from build123d import *
from OCP.BRepFilletAPI import BRepFilletAPI_MakeChamfer

# Parameters (mm, degrees)
EXTRUDE_1_DEPTH     = 21.3
CUT_EXTRUDE_1_DEPTH = 42.6
FILLET_1_R          = 3
CHAMFER_1_SIZE      = 1
CHAMFER_1_SIZE2     = 0.839099631


with BuildPart() as part:
    # Эскиз1 → Бобышка-Вытянуть1 (new, symmetric)
    with BuildSketch(Plane(origin=(0, 0, 0), x_dir=(1, 0, 0), z_dir=(0, 1, 0))):
        Polygon((0, 0), (25.3, 0), (25.3, 3.3), (3.3, 3.3), (3.3, 35.5), (0, 35.5), align=None)
    extrude(amount=EXTRUDE_1_DEPTH, both=True)

    # Эскиз2 → Вырез-Вытянуть1 (cut)
    with BuildSketch(Plane.XY):
        with BuildLine():
            Line((17.3, 13), (13.3, 13))
            ThreePointArc((13.3, 13), (10.3, 16), (13.3, 19))
            Line((13.3, 19), (17.3, 19))
            ThreePointArc((17.3, 19), (20.3, 16), (17.3, 13))
        make_face()
        with BuildLine():
            Line((17.3, -3.022560491), (13.3, -3.022560491))
            ThreePointArc((13.3, -3.022560491), (10.277439509, 0), (13.3, 3.022560491))
            Line((13.3, 3.022560491), (17.3, 3.022560491))
            ThreePointArc((17.3, 3.022560491), (20.322560491, 0), (17.3, -3.022560491))
        make_face()
        with BuildLine():
            Line((17.3, -19.150761356), (13.3, -19.150761356))
            ThreePointArc((13.3, -19.150761356), (10.149238644, -16), (13.3, -12.849238644))
            Line((13.3, -12.849238644), (17.3, -12.849238644))
            ThreePointArc((17.3, -12.849238644), (20.450761356, -16), (17.3, -19.150761356))
        make_face()
    extrude(amount=-CUT_EXTRUDE_1_DEPTH, mode=Mode.SUBTRACT)

    # Скругление1
    fillet_1_edges = [part.edges().sort_by_distance(p)[0] for p in [
        (25.3, 21.3, -1.65),
        (1.65, 21.3, -35.5),
        (1.65, -21.3, -35.5),
        (25.3, -21.3, -1.65),
    ]]
    fillet(fillet_1_edges, radius=FILLET_1_R)

    # Фаска1: one chamfer whose edges measure the first distance from different faces: ONE call of the kernel's chamfer builder (chamfer() names one face for all edges)
    chamfer_1_edges_1 = [part.edges().sort_by_distance(p)[0] for p in [
        (24.421320344, -20.421320344, 0),
        (11.15, -21.3, 0),
        (11.15, 21.3, 0),
        (25.3, 0, 0),
        (24.421320344, 20.421320344, 0),
    ]]
    chamfer_1_side_1 = [part.faces().sort_by_distance(p)[0] for p in [
        (11.15, -20.804535571, 0),
    ]]
    chamfer_1_edges_2 = [part.edges().sort_by_distance(p)[0] for p in [
        (3.3, 21.3, -17.9),
        (3.3, -21.3, -17.9),
        (3.3, 0, -35.5),
        (3.3, 20.421320344, -34.621320344),
        (3.3, -20.421320344, -34.621320344),
    ]]
    chamfer_1_side_2 = [part.faces().sort_by_distance(p)[0] for p in [
        (3.3, 0, -19.356425923),
    ]]
    chamfer_1_edges_3 = [part.edges().sort_by_distance(p)[0] for p in [
        (0, 0, -35.5),
        (0, -21.3, -16.25),
        (0, 21.3, -16.25),
        (0, 20.421320344, -34.621320344),
        (0, -20.421320344, -34.621320344),
    ]]
    chamfer_1_side_3 = [part.faces().sort_by_distance(p)[0] for p in [
        (0, 0, -17.706261494),
    ]]
    chamfer_1_edges_4 = [part.edges().sort_by_distance(p)[0] for p in [
        (12.8, -21.3, -3.3),
        (12.8, 21.3, -3.3),
        (25.3, 0, -3.3),
        (24.421320344, 20.421320344, -3.3),
        (24.421320344, -20.421320344, -3.3),
    ]]
    chamfer_1_side_4 = [part.faces().sort_by_distance(p)[0] for p in [
        (24.820546144, 0, -3.3),
    ]]
    chamfer_1 = BRepFilletAPI_MakeChamfer(part.part.solid().wrapped)
    for e in chamfer_1_edges_1:
        chamfer_1.Add(CHAMFER_1_SIZE, CHAMFER_1_SIZE2, e.wrapped, chamfer_1_side_1[0].wrapped)  # the first distance lies on this face
    for e in chamfer_1_edges_2:
        chamfer_1.Add(CHAMFER_1_SIZE, CHAMFER_1_SIZE2, e.wrapped, chamfer_1_side_2[0].wrapped)  # the first distance lies on this face
    for e in chamfer_1_edges_3:
        chamfer_1.Add(CHAMFER_1_SIZE, CHAMFER_1_SIZE2, e.wrapped, chamfer_1_side_3[0].wrapped)  # the first distance lies on this face
    for e in chamfer_1_edges_4:
        chamfer_1.Add(CHAMFER_1_SIZE, CHAMFER_1_SIZE2, e.wrapped, chamfer_1_side_4[0].wrapped)  # the first distance lies on this face
    add(Compound.cast(chamfer_1.Shape()), mode=Mode.REPLACE)


solid = part.part
Source: CAD feature listing. Evaluate the final solid. Frame: model axes, mm. A direction names the side the tool comes from. Give positions to 0.01 mm unless a question says otherwise; leave off trailing zeros. Order: outer loops, then holes, each group sorted by start corner. A loop starts at its lowest first (then second) coordinate and runs counter-clockwise, first axis right, second up. Notation, with made-up numbers: (76, 83.5) -> (116, 83.5) arc R16 ccw to (116, 102.5) -> close; hole circle Ø10 at (78.25, 23.5). An arc over 180 degrees is marked (long way). Use a Markdown table: item, result.
1) Section query D-D, the plane y = -9. Return the cut outline in (x, z), then the cut area to 3 significant figures.
Answer list:
| item | result |
|---|---|
| outline | (0, -34.5) -> (0.84, -35.5) -> (2.46, -35.5) -> (3.3, -34.5) -> (3.3, -3.3) -> (24.3, -3.3) -> (25.3, -2.46) -> (25.3, -0.84) -> (24.3, 0) -> (0, 0) -> close |
| area | 188 mm² |
2) Contact query for flat-ended pins moving along their axis: P1, Ø1, axis at x = 3, y = -15, coming from the -Z side; P2, Ø4, axis at x = 16.5, y = -8.5, coming from the -Z side; P3, Ø12, axis at y = -11.5, z = -28, coming from the +X side. Output: stop coordinate, or through.
Answer list:
| item | result |
|---|---|
| P1 | z = -35.45 |
| P2 | z = -3.3 |
| P3 | x = 3.3 |
3) Section query A-A, the plane y = -16. Return the cut outline in (x, z).
Answer list:
| item | result |
|---|---|
| outline | (0, -34.5) -> (0.84, -35.5) -> (2.46, -35.5) -> (3.3, -34.5) -> (3.3, -3.3) -> (10.15, -3.3) -> (10.15, 0) -> (0, 0) -> close; (20.45, -3.3) -> (24.3, -3.3) -> (25.3, -2.46) -> (25.3, -0.84) -> (24.3, 0) -> (20.45, 0) -> close |
4) Mould query, pull axis Y, two halves, no side actions, for faces 5 (the flat face through (25.3, 0, -2)), 6 (the cylindrical face through (20.3, 16.1, -1.6)), 7 (the flat face through (0.43, -20.81, -16.48)), 8 (the conical face through (0.332, 20.013, -34.175)). Classes: +Y half, -Y half, draft (parallel to the pull), parting line (faces both ways), or undercut.
Answer list:
| item | result |
|---|---|
| face 5 | draft |
| face 6 | undercut |
| face 7 | -Y half |
| face 8 | +Y half |
5) Section query C-C, the plane y = 0. Return the cut outline in (x, z), then the cut area to 3 significant figures.
Answer list:
| item | result |
|---|---|
| outline | (0, -34.5) -> (0.84, -35.5) -> (2.46, -35.5) -> (3.3, -34.5) -> (3.3, -3.3) -> (10.28, -3.3) -> (10.28, 0) -> (0, 0) -> close; (20.32, -3.3) -> (24.3, -3.3) -> (25.3, -2.46) -> (25.3, -0.84) -> (24.3, 0) -> (20.32, 0) -> close |
| area | 155 mm² |
6) Ray query, line 1 along Z through (x, y) = (10.25, 3.5); line 2 along X through (y, z) = (5, -7); line 3 along Y through (x, z) = (3.25, -10). Return the intervals inside material, ascending. Write a range as [from, to].
Answer list:
| item | result |
|---|---|
| line 1 | [-3.3, 0] |
| line 2 | [0, 3.3] |
| line 3 | [-20.36, 20.36] |
7) Reachability of faces 1 (the flat face through (2.87, -20.81, -17.69)), 2 (the flat face through (15, -3.023, -2)), 3 (the flat face through (3.3, 0, -19)), 4 (the conical face through (23.975, -20.013, -0.332)) from +Z, -Z, +X, -X, +Y, -Y: full face, straight path, thin tool, end or side. Return the list, or none.
Answer list:
| item | result |
|---|---|
| face 1 | -Z, +X, -Y |
| face 2 | +Z, -Z |
| face 3 | -Z, +X, +Y, -Y |
| face 4 | +Z, +X, -Y |
8) Section query B-B, the plane z = -9. Return the cut outline in (x, y).
Answer list:
| item | result |
|---|---|
| outline | (0, -20.3) -> (0.84, -21.3) -> (2.46, -21.3) -> (3.3, -20.3) -> (3.3, 20.3) -> (2.46, 21.3) -> (0.84, 21.3) -> (0, 20.3) -> close |
